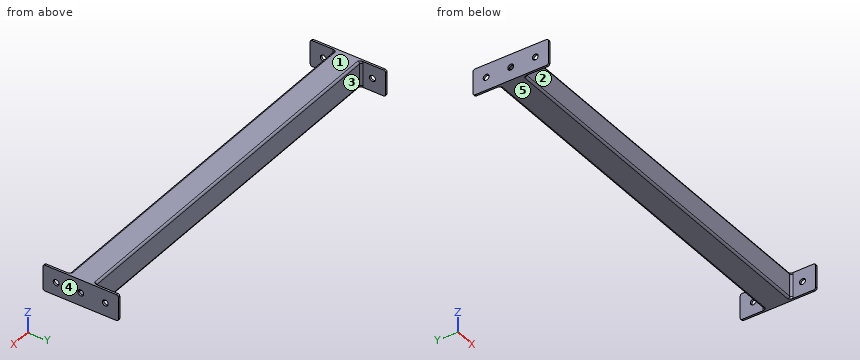
```python
from build123d import *

# Parameters (mm, degrees)
SKETCH1_W           = 40
SKETCH1_H           = 40
SKETCH1_W_2         = 34
SKETCH1_H_2         = 34
BOSS_EXTRUDE1_DEPTH = 289.5
FILLET1_R           = 1
FILLET2_R           = 3
SKETCH2_W           = 40
SKETCH2_H           = 115
SKETCH2_R           = 4.5
BOSS_EXTRUDE2_DEPTH = 3
FILLET3_R           = 3
FILLET4_R           = 3


with BuildPart() as part:
    # Sketch1 → Boss-Extrude1 (new body)
    with BuildSketch(Plane(origin=(0, 0, 0), x_dir=(0, 0, -1), z_dir=(1, 0, 0))):
        Rectangle(SKETCH1_W, SKETCH1_H)
        Rectangle(SKETCH1_W_2, SKETCH1_H_2, mode=Mode.SUBTRACT)
    extrude(amount=BOSS_EXTRUDE1_DEPTH)

    # Fillet1
    fillet1_edges = [part.edges().sort_by_distance(p)[0] for p in [
        (144.75, -17, -17),
        (144.75, 17, -17),
        (144.75, 17, 17),
        (144.75, -17, 17),
    ]]
    fillet(fillet1_edges, radius=FILLET1_R)

    # Fillet2
    fillet2_edges = [part.edges().sort_by_distance(p)[0] for p in [
        (144.75, -20, -20),
        (144.75, -20, 20),
        (144.75, 20, 20),
        (144.75, 20, -20),
    ]]
    fillet(fillet2_edges, radius=FILLET2_R)

    # Sketch2 → Boss-Extrude2 (add)
    with BuildSketch(Plane(origin=(289.5, 0, 0), x_dir=(0, 0, -1), z_dir=(1, 0, 0))):
        Rectangle(SKETCH2_W, SKETCH2_H)
        Circle(SKETCH2_R, mode=Mode.SUBTRACT)
        with Locations((0, -37.5)):
            Circle(SKETCH2_R, mode=Mode.SUBTRACT)
        with Locations((0, 37.5)):
            Circle(SKETCH2_R, mode=Mode.SUBTRACT)
    extrude(amount=BOSS_EXTRUDE2_DEPTH)

    # Fillet3
    # the kernel refuses this fillet: 3 mm, written as the material it adds along each edge
    with BuildSketch(Plane(origin=(289.5, -20, 17), x_dir=(0, -1, 0), z_dir=(0, 0, -1)), Plane(origin=(289.5, 20, -17), x_dir=(0, 1, 0), z_dir=(0, 0, 1))) as fillet3_piece_1:
        with BuildLine():
            CenterArc((FILLET3_R, FILLET3_R), FILLET3_R, 180, 90)
            Line((0, FILLET3_R), (0, 0))
            Line((0, 0), (FILLET3_R, 0))
        make_face()
    extrude(amount=34)
    with BuildSketch(Plane(origin=(289.5, 17, 17), x_dir=(0, 1, 0), z_dir=(0, 0, -1))) as fillet3_piece_2_section:
        with BuildLine():
            CenterArc((3 + FILLET3_R, -FILLET3_R), FILLET3_R, 90, 90)
            Line((3, -FILLET3_R), (3, 0))
            Line((3, 0), (3 + FILLET3_R, 0))
        make_face()
    fillet3_piece_2 = revolve(axis=Axis((289.5, 17, 17), (1, 0, 0)), revolution_arc=233.296989237, mode=Mode.PRIVATE)
    fillet3_piece_2 = split(fillet3_piece_2, bisect_by=Plane(origin=(288.998099396, 20.659325751, 20), z_dir=(0, 0, -1)), keep=Keep.TOP, mode=Mode.PRIVATE)
    fillet3_piece_2 = split(fillet3_piece_2, bisect_by=Plane(origin=(288.998099396, 20.659325751, 17), z_dir=(0, 0, 1)), keep=Keep.TOP, mode=Mode.PRIVATE)
    add(fillet3_piece_2)
    with BuildSketch(Plane(origin=(289.5, 17, -17), x_dir=(0, -0.5976672776328276, 0.8017442392976482), z_dir=(0, 0.8017442392976482, 0.5976672776328276))) as fillet3_piece_3_section:
        with BuildLine():
            CenterArc((3 + FILLET3_R, -FILLET3_R), FILLET3_R, 90, 90)
            Line((3, -FILLET3_R), (3, 0))
            Line((3, 0), (3 + FILLET3_R, 0))
        make_face()
    fillet3_piece_3 = revolve(axis=Axis((289.5, 17, -17), (1, 0, 0)), revolution_arc=233.296989237, mode=Mode.PRIVATE)
    fillet3_piece_3 = split(fillet3_piece_3, bisect_by=Plane(origin=(288.565115083, 19.249816872, -20), z_dir=(0, 0, 1)), keep=Keep.TOP, mode=Mode.PRIVATE)
    fillet3_piece_3 = split(fillet3_piece_3, bisect_by=Plane(origin=(288.565115083, 19.249816872, -17), z_dir=(0, 0, -1)), keep=Keep.TOP, mode=Mode.PRIVATE)
    add(fillet3_piece_3)
    with BuildSketch(Plane(origin=(289.5, -17, -17), x_dir=(0, -1, 0), z_dir=(0, 0, 1))) as fillet3_piece_4_section:
        with BuildLine():
            CenterArc((3 + FILLET3_R, -FILLET3_R), FILLET3_R, 90, 90)
            Line((3, -FILLET3_R), (3, 0))
            Line((3, 0), (3 + FILLET3_R, 0))
        make_face()
    fillet3_piece_4 = revolve(axis=Axis((289.5, -17, -17), (1, 0, 0)), revolution_arc=233.296989237, mode=Mode.PRIVATE)
    fillet3_piece_4 = split(fillet3_piece_4, bisect_by=Plane(origin=(288.998099396, -20.659325751, -20), z_dir=(0, 0, 1)), keep=Keep.TOP, mode=Mode.PRIVATE)
    fillet3_piece_4 = split(fillet3_piece_4, bisect_by=Plane(origin=(288.998099396, -20.659325751, -17), z_dir=(0, 0, -1)), keep=Keep.TOP, mode=Mode.PRIVATE)
    add(fillet3_piece_4)
    with BuildSketch(Plane(origin=(289.5, -17, 17), x_dir=(0, -1, 0), z_dir=(0, 0, -1))) as fillet3_piece_5_section:
        with BuildLine():
            CenterArc((3 + FILLET3_R, FILLET3_R), FILLET3_R, 180, 90)
            Line((3, FILLET3_R), (3, 0))
            Line((3, 0), (3 + FILLET3_R, 0))
        make_face()
    fillet3_piece_5 = revolve(axis=Axis((289.5, -17, 17), (-1, 0, 0)), revolution_arc=233.296989237, mode=Mode.PRIVATE)
    fillet3_piece_5 = split(fillet3_piece_5, bisect_by=Plane(origin=(288.998099366, -20.659325736, 20), z_dir=(0, 0, -1)), keep=Keep.TOP, mode=Mode.PRIVATE)
    fillet3_piece_5 = split(fillet3_piece_5, bisect_by=Plane(origin=(288.998099366, -20.659325736, 17), z_dir=(0, 0, 1)), keep=Keep.TOP, mode=Mode.PRIVATE)
    add(fillet3_piece_5)

    # Fillet4
    fillet4_edges = [part.edges().sort_by_distance(p)[0] for p in [
        (291, -57.5, -20),
        (291, 57.5, -20),
        (291, 57.5, 20),
        (291, -57.5, 20),
    ]]
    fillet(fillet4_edges, radius=FILLET4_R)

    # Mirror1: part across plane


with BuildPart() as part_1:
    add(part.part)
    add(part.part.mirror(Plane(origin=(0, 0, 0), x_dir=(0, 0, 1), z_dir=(1, 0, 0))))


solid = part_1.part
```
Geometry: final body of the model. Coordinates: model frame, mm. Face numbers are marked on the shaded views. A direction names the side the tool comes from. Round coordinates to 2 decimals unless told otherwise and drop trailing zeros. Write each loop counter-clockwise with the first axis right and the second up, starting at its lowest first coordinate (ties: lowest second). Pieces come first, ordered by that corner, then holes.
Item 1: Section query B-B (y = -9.5). Return loops of the section in (x, z).
Item 2: Section query C-C (z = 10.5). Return loops of the section in (x, y), plus the area to 3 significant figures.
Item 3: Material intervals for L1, parallel to Y at x = -291.5, z = 0; L2, parallel to Y at x = -74, z = 0.5; L3, parallel to X at y = -49, z = 17, sorted ascending.
Item 4: Set-up query: the marked faces 1 and 2. Return all of +Z, -Z, +X, -X, +Y, -Y with unobstructed straight access to the full face (end or side cutting, diameter ignored); none if empty.
Item 5: Section query A-A (x = 80.5). Return loops of the section in (y, z), plus the area to 3 significant figures.
Item 6: Mould query, pull axis X, two halves, no side actions, for the marked faces 3, 4 and 5. Classes: +X half, -X half, draft (parallel to the pull), parting line (faces both ways), or undercut.
Item 7: Pin query (flat end, axial travel): P1, Ø10, axis at x = 84, z = 5, coming from the -Y side; P2, Ø1.5, axis at x = -185, z = 4, coming from the +Y side. Return the tip coordinate at first contact, or that it passes through.
Completed:
1. outline: (-292.5, -20) - (292.5, -20) - (292.5, 20) - (-292.5, 20) - close; hole (-289.5, -17) - (289.5, -17) - (289.5, 17) - (-289.5, 17) - close
2. outline: (-292.5, -57.5) - (-289.5, -57.5) - (-289.5, -23) arc R3 cw to (-286.5, -20) - (286.5, -20) arc R3 cw to (289.5, -23) - (289.5, -57.5) - (292.5, -57.5) - (292.5, 57.5) - (289.5, 57.5) - (289.5, 23) arc R3 cw to (286.5, 20) - (-286.5, 20) arc R3 cw to (-289.5, 23) - (-289.5, 57.5) - (-292.5, 57.5) - close; hole (-289.5, -17) - (289.5, -17) - (289.5, 17) - (-289.5, 17) - close
2. area: 4,170 mm2
3. L1: y = -57.5 to -42, -33 to -4.5, 4.5 to 33, 42 to 57.5
3. L2: y = -20 to -17, 17 to 20
3. L3: x = -292.5 to -289.5, 289.5 to 292.5
4. face 1: +Z, +X, -X, +Y, -Y
4. face 2: +Z, -Z, -Y
5. outline: (-20, -17) arc R3 ccw to (-17, -20) - (17, -20) arc R3 ccw to (20, -17) - (20, 17) arc R3 ccw to (17, 20) - (-17, 20) arc R3 ccw to (-20, 17) - close; hole (-17, -16) arc R1 ccw to (-16, -17) - (16, -17) arc R1 ccw to (17, -16) - (17, 16) arc R1 ccw to (16, 17) - (-16, 17) arc R1 ccw to (-17, 16) - close
5. area: 437 mm2
6. face 3: undercut
6. face 4: +X half
6. face 5: draft
7. P1: stops at y = -20
7. P2: stops at y = 20
